from build123d import *

# Parameters (mm, degrees)
FILLET1_R       = 0.2
RECPAT_COUNT    = 2
RECPAT_ANGLE    = 90
THDSCHPAT_COUNT = 8
THDSCHPAT_PITCH = 0.657142857


with BuildPart() as part:
    # BodySke → Base-Revolve (revolve)
    with BuildSketch(Plane.XY, mode=Mode.PRIVATE) as base_revolve_sk:
        Polygon((3.05, 2), (3.05, 5), (2.05, 5), (2.05, 0), (9.05, 0), (9.05, 2), align=None)
    revolve(base_revolve_sk.sketch.rotate(Axis((-6.35, 0, 0), (1, 0, 0)), 90), axis=Axis((-6.35, 0, 0), (1, 0, 0)))

    # Fillet1
    fillet1_edges = [part.edges().sort_by_distance(p)[0] for p in [
        (3.05, 0, -2),
    ]]
    fillet(fillet1_edges, radius=FILLET1_R)

    # PanSke → Pan (revolve)
    with BuildSketch(Plane.XY):
        with BuildLine():
            Line((2.05, 4.424646879), (2.05, 0))
            Line((2.05, 0), (0, 0))
            ThreePointArc((0, 0), (0.537396082, 2.438237068), (2.05, 4.424646879))
        make_face()
    revolve(axis=Axis((0, 0, 0), (1, 0, 0)))

    # Sketch3 → Recess section 0
    with BuildSketch(Plane(origin=(0, 0, 0), x_dir=(0, 0, -1), z_dir=(1, 0, 0))):
        with BuildLine():
            Line((-0.515, 2.15), (0.515, 2.15))
            Line((0.515, 2.15), (0.515, -2.15))
            Line((0.515, -2.15), (-0.515, -2.15))
            Line((-0.515, -2.15), (-0.515, 2.15))
        make_face()
    # Sketch4 → Recess section 1
    with BuildSketch(Plane(origin=(2.34, 0, 0), x_dir=(0, 0, -1), z_dir=(1, 0, 0))):
        with BuildLine():
            Line((-0.515, 2.106524682), (0.515, 2.106524682))
            Line((0.515, 2.106524682), (0.515, -2.106524682))
            Line((0.515, -2.106524682), (-0.515, -2.106524682))
            Line((-0.515, -2.106524682), (-0.515, 2.106524682))
        make_face()
    recess = loft(mode=Mode.SUBTRACT)

    # RecPat: Recess ×2 about axis
    recpat_axis = Axis((0, 0, 0), (1, 0, 0))
    for i in range(1, RECPAT_COUNT):
        add(recess.rotate(recpat_axis, i * RECPAT_ANGLE / (RECPAT_COUNT - 1)), mode=Mode.SUBTRACT)

    # RecCorSke → RecessCore (revolve, cut)
    with BuildSketch(Plane.XY, mode=Mode.PRIVATE) as recesscore_sk:
        Polygon((0, 0), (0, 1.172663335), (4.6, 0.851), (4.876506661, 0), align=None)
    revolve(recesscore_sk.sketch.rotate(Axis((-3.175, 0, 0), (1, 0, 0)), 90), axis=Axis((-3.175, 0, 0), (1, 0, 0)), mode=Mode.SUBTRACT)

    # ThdSchSke → ThreadSchematic (revolve, cut)
    with BuildSketch(Plane.XY, mode=Mode.PRIVATE) as threadschematic_sk:
        Polygon((4.45, -1.61), (4.17691906, -2), (4.17691906, -2.5), (4.72308094, -2.5), (4.72308094, -2), align=None)
    threadschematic = revolve(threadschematic_sk.sketch.rotate(Axis((-3.175, 0, 0), (1, 0, 0)), 270), axis=Axis((-3.175, 0, 0), (1, 0, 0)), mode=Mode.SUBTRACT)

    # ThdSchPat: ThreadSchematic ×8
    with Locations(*[(i * THDSCHPAT_PITCH, 0, 0) for i in range(1, THDSCHPAT_COUNT)]):
        add(threadschematic, mode=Mode.SUBTRACT)


solid = part.part
Part model, mm, in its own coordinate system. A direction names the side the tool comes from. Give positions to 0.01 mm unless a question says otherwise; leave off trailing zeros. Loops run counter-clockwise (first coordinate to the right, second up) from the corner with the lowest first, then second, coordinate; pieces in that order, holes last.
(1) Pin check, flat tips, straight feed: pin 1 (1.5 mm diameter, centred on y = -3, z = 0, fed in from -X); pin 2 (1.5 mm diameter, centred on x = 5, y = -1, fed in from -Z); pin 3 (0.8 mm diameter, centred on y = -1.5, z = 0, fed in from -X). Stop position of each tip, or through.
Return value:
pin 1: stops at x = 0.45
pin 2: stops at z = -1.98
pin 3: stops at x = 2.34
(2) Band-saw the part on A-A (z = -2.5). Write the cut outline in (x, y), and give its area (3 significant figures).
Return value:
outline: (2.05, -4.33) - (3.05, -4.33) - (3.05, 4.33) - (2.05, 4.33) - (2.05, 3.65) arc R5.23 ccw to (2.05, -3.65) - close
area: 16.1 mm2
(3) Drill centre lines: line 1 along X through (y, z) = (-4, -2.5); line 2 along Z through (x, y) = (4.5, -0.5); line 3 along Y through (x, z) = (1.5, -1) (3 decimals). Where is each one in solid material? Low to high.
Return value:
line 1: x = 2.05 to 3.05
line 2: z = -1.61 to -0.7, 0.7 to 1.61
line 3: y = -3.762 to -0.515, 0.515 to 3.762
(4) Band-saw the part on C-C (y = -3.25). Write the cut outline in (x, z).
Return value:
outline: (2.05, -3.8) - (3.05, -3.8) - (3.05, 3.8) - (2.05, 3.8) - (2.05, 3) arc R4.8 ccw to (2.05, -3) - close
(5) Pull direction X, two halves, no side cores. Call faces 3 (the flat face through (9.05, 0, 0)), 4 (the flat face through (2.34, 0, -1.5)): pulls with the +X half, pulls with the -X half, needs draft (parallel to the pull), parting line crosses it, or undercut.
Return value:
face 3: pulls with the +X half
face 4: pulls with the -X half
(6) 3-axis set-ups, long thin cutter, end or side, ignore diameter. For faces 1 (the flat face through (3.05, 1, -2.2)), 2 (the flat face through (2.34, 1.5, 0)): which of +Z, -Z, +X, -X, +Y, -Y reach the whole face in a straight line?
Return value:
face 1: +X
face 2: -X
(7) Band-saw the part on B-B (y = 1.75). Count the separate pieces of the cut face and the enclosed holes in it, and give its area (3 significant figures).
Return value:
separate pieces: 8
enclosed holes: 0
area: 24.3 mm2
